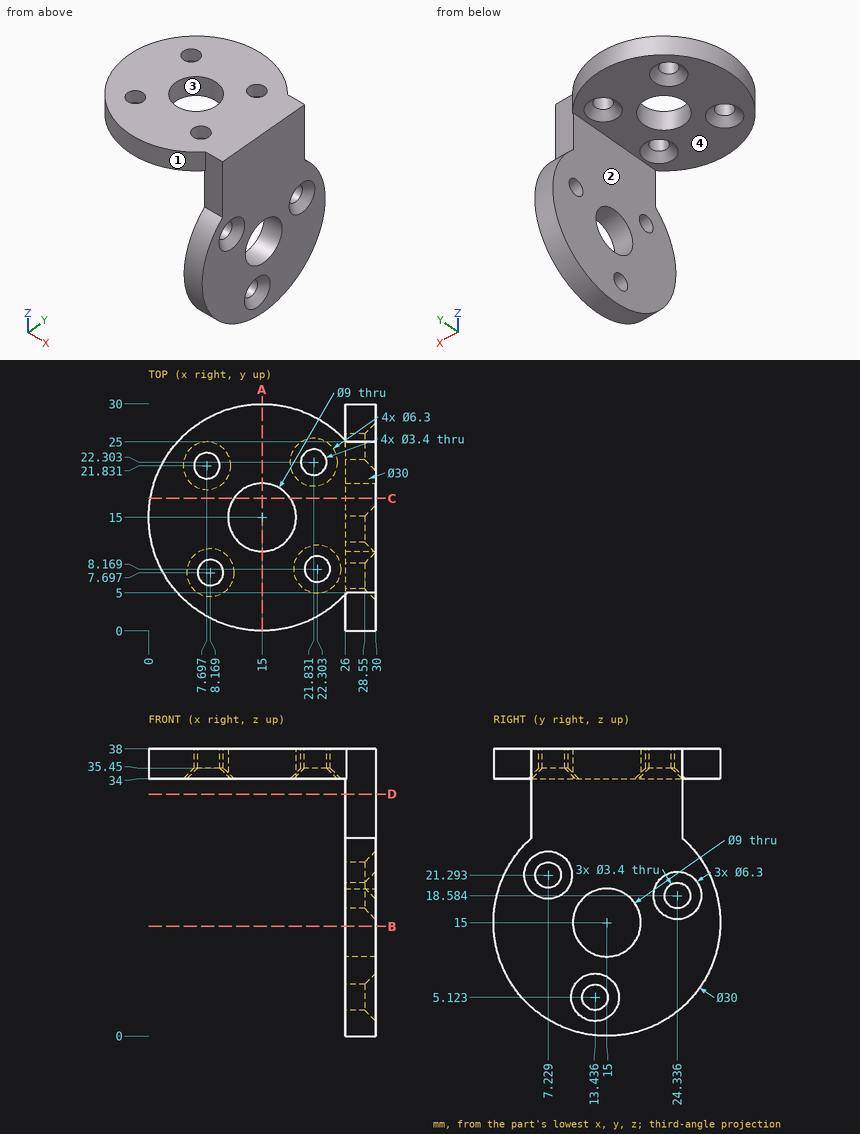
Geometry: see drawing. Coordinates: mm, zero at the bounding-box minimum. Coordinates: 2 decimals unless noted, no trailing zeros. Loops run counter-clockwise (first coordinate to the right, second up) from the corner with the lowest first, then second, coordinate; pieces in that order, holes last. Notation, with made-up numbers: M 27,64 L 47,64 A20 ccw 47,94 Z; hole C -38.5,51.25 d5. An arc over 180 degrees is marked long. Put each result on its own line as item: value. Start each with the question number.
1) Ray query, L1, parallel to Y at x = 15, z = 36.4; L2, parallel to Z at x = 29.1, y = 15 (1 decimal); L3, parallel to X at y = 20.5, z = 16.5. Return the intervals inside material, ascending. Write a range as from..to.
2) Cut plane C-C on y = 17.5. Return the cut outline in (x, z).
3) Pull-direction query (X, two-part tool) for the marked faces 1, 2, 3 and 4; classes: pulls with the +X half, pulls with the -X half, needs draft (parallel to the pull), parting line crosses it, or undercut.
4) Contact query for flat-ended pins moving along their axis: pin 1 Ø14.5 at (y, z) = (15, 15) entering from -X; pin 2 Ø2 at (x, y) = (8.17, 7.7) entering from +Z; pin 3 Ø3 at (x, z) = (29, 33.5) entering from -Y; pin 4 Ø10 at (x, y) = (25, 6) entering from -Z. Output: stop coordinate, or through.
5) Cut plane D-D on z = 32. Return the cut outline in (x, y).
6) Cut plane A-A on x = 15. Return the cut outline in (y, z).
7) Cut plane B-B on z = 14.5. Return the cut outline in (x, y).
The answers:
1. L1: y = 0..10.5, 19.5..30
1. L2: z = 0..3.5, 6.7..10.5, 19.5..38
1. L3: x = 26..30
2. outline: M 0.21,34 L 11.26,34 L 11.26,38 L 0.21,38 Z; M 18.74,34 L 26,34 L 26,18.74 L 30,18.74 L 30,38 L 18.74,38 Z; M 26,0.21 L 30,0.21 L 30,11.26 L 26,11.26 Z
3. face 1: parting line crosses it
3. face 2: pulls with the -X half
3. face 3: undercut
3. face 4: needs draft
4. pin 1: stops at x = 26
4. pin 2: passes through
4. pin 3: stops at y = 5
4. pin 4: stops at z = 0.57
5. outline: M 26,5 L 30,5 L 30,25 L 26,25 Z
6. outline: M 0,34 L 10.5,34 L 10.5,38 L 0,38 Z; M 19.5,34 L 30,34 L 30,38 L 19.5,38 Z
7. outline: M 26,0.01 L 30,0.01 L 30,10.53 L 26,10.53 Z; M 26,19.47 L 30,19.47 L 30,29.99 L 26,29.99 Z
